from build123d import *

# Parameters (mm, degrees)
SKETCH_1_W             = 140
SKETCH_1_H             = 64
SM_BASE_FLANGE_1_DEPTH = 1
FILLET_1_R             = 5
SKETCH_4_R             = 2
CUT_EXTRUDE_2_DEPTH    = 10
SKETCH_5_R             = 13.6
SKETCH_5_R_2           = 1.5
CUT_EXTRUDE_3_DEPTH    = 10


# Sheet-metal steps are written as plain solids
with BuildPart() as part:
    # Sketch 1 → Базовая кромка1 (new body)
    with BuildSketch(Plane(origin=(0, 0, 0), x_dir=(1, 0, 0), z_dir=(0, 1, 0))):
        with Locations((16.228693113, 2.194635649)):
            Rectangle(SKETCH_1_W, SKETCH_1_H)
    extrude(amount=-SM_BASE_FLANGE_1_DEPTH)

    # Скругление1
    fillet_1_edges = [part.edges().sort_by_distance(p)[0] for p in [
        (-53.771306887, -0.5, -34.194635649),
        (86.228693113, -0.5, -34.194635649),
        (86.228693113, -0.5, 29.805364351),
        (-53.771306887, -0.5, 29.805364351),
    ]]
    fillet(fillet_1_edges, radius=FILLET_1_R)

    # Эскиз4 → Вырез-Вытянуть2 (cut)
    with BuildSketch(Plane(origin=(0, 0, 0), x_dir=(1, 0, 0), z_dir=(0, 1, 0))):
        with Locations(Location((-48.771306887, 29.194635649, 0), (0, 0, 270))):
            Circle(SKETCH_4_R)
        with Locations(Location((81.228693113, 29.194635649, 0), (0, 0, 270))):
            Circle(SKETCH_4_R)
        with Locations(Location((-48.771306887, -24.805364351, 0), (0, 0, 270))):
            Circle(SKETCH_4_R)
        with Locations(Location((81.228693113, -24.805364351, 0), (0, 0, 270))):
            Circle(SKETCH_4_R)
    extrude(amount=-CUT_EXTRUDE_2_DEPTH, mode=Mode.SUBTRACT)

    # Эскиз5 → Вырез-Вытянуть3 (cut)
    with BuildSketch(Plane(origin=(0, 0, 0), x_dir=(1, 0, 0), z_dir=(0, 1, 0))):
        with Locations(Location((-6.271306887, 2.194635649, 0), (0, 0, 270))):
            Circle(SKETCH_5_R)
        with Locations(Location((38.728693113, 2.194635649, 0), (0, 0, 270))):
            Circle(SKETCH_5_R)
        with Locations(Location((-19.271306887, 15.194635649, 0), (0, 0, 270))):
            Circle(SKETCH_5_R_2)
        with Locations(Location((6.728693113, 15.194635649, 0), (0, 0, 270))):
            Circle(SKETCH_5_R_2)
        with Locations(Location((-19.271306887, -10.805364351, 0), (0, 0, 270))):
            Circle(SKETCH_5_R_2)
        with Locations(Location((6.728693113, -10.805364351, 0), (0, 0, 270))):
            Circle(SKETCH_5_R_2)
        with Locations(Location((25.728693113, 15.194635649, 0), (0, 0, 270))):
            Circle(SKETCH_5_R_2)
        with Locations(Location((51.728693113, 15.194635649, 0), (0, 0, 270))):
            Circle(SKETCH_5_R_2)
        with Locations(Location((25.728693113, -10.805364351, 0), (0, 0, 270))):
            Circle(SKETCH_5_R_2)
        with Locations(Location((51.728693113, -10.805364351, 0), (0, 0, 270))):
            Circle(SKETCH_5_R_2)
    extrude(amount=-CUT_EXTRUDE_3_DEPTH, mode=Mode.SUBTRACT)


solid = part.part
Geometry: final body of the model. Coordinates: model frame, mm. Coordinates: 2 decimals unless noted, no trailing zeros. Loops run counter-clockwise (first coordinate to the right, second up) from the corner with the lowest first, then second, coordinate; pieces in that order, holes last. Notation, with made-up numbers: M 83,84 L 123,84 A11 cw 123,88 Z; hole C 45.5,55 d9. An arc over 180 degrees is marked long. One line per item, written item: value. Start each with the question number.
1) Cut plane A-A (x = 29). Return loops of the section in (y, z), then the cut area to 3 significant figures.
2) Material intervals for L1, parallel to X at y = -0.55, z = -29.5; L2, parallel to X at y = -0.7, z = 25; L3, parallel to Z at x = -7, y = -0.6, sorted ascending. Write a range as from..to.
3) Pin query (flat end, axial travel): P1, Ø10, axis at x = 64, z = -27, coming from the +Y side. Return the tip coordinate at first contact, or that it passes through.
4) Cut plane D-D (x = -11.5). Return loops of the section in (y, z).
5) Cut plane C-C (y = -0.2). Count the separate pieces of the cut face and the enclosed holes in it, then the cut area to 3 significant figures.
6) Draft query along Z for faces 1 (the cylindrical face through (84.803, -0.507, -32.691)), 2 (the cylindrical face through (8, -0.5, -14.4)), 3 (the cylindrical face through (84.725, -0.507, 28.38)). Return one class per face: released by +Z, released by -Z, zero draft, split by the parting line, or undercut.
7) Cut plane B-B (z = -2.5). Return loops of the section in (x, y), then the cut area to 3 significant figures.
Evaluation:
1. outline: M -1,-34.19 L 0,-34.19 L 0,-11.7 L -1,-11.7 Z; M -1,7.31 L 0,7.31 L 0,29.81 L -1,29.81 Z
1. area: 45.0 mm^2
2. L1: -53.76..-50.75, -46.79..79.25, 83.21..86.22
2. L2: -53.77..-50.76, -46.78..79.24, 83.22..86.22
2. L3: -34.19..-15.78, 11.39..29.81
3. P1: y = 0
4. outline: M -1,-34.19 L 0,-34.19 L 0,-14.75 L -1,-14.75 Z; M -1,10.36 L 0,10.36 L 0,29.81 L -1,29.81 Z
5. separate pieces: 1
5. enclosed holes: 14
5. area: 7,670 mm^2
6. face 1: released by -Z
6. face 2: undercut
6. face 3: released by +Z
7. outline: M -53.77,-1 L -19.87,-1 L -19.87,0 L -53.77,0 Z; M 7.33,-1 L 25.13,-1 L 25.13,0 L 7.33,0 Z; M 52.33,-1 L 86.23,-1 L 86.23,0 L 52.33,0 Z
7. area: 85.6 mm^2
